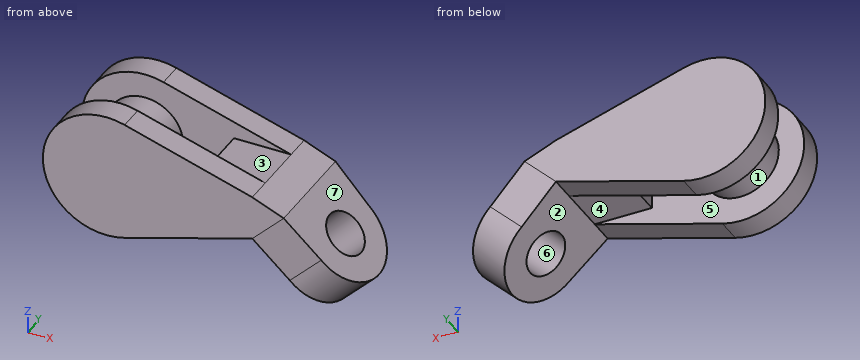
from build123d import *

# Parameters (mm, degrees)
BOSS_EXTRUDE1_DEPTH             = 35
BOSS_EXTRUDE2_START             = -40
BOSS_EXTRUDE2_DEPTH             = 80
SKETCH7_R                       = 17.5
BOSS_EXTRUDE8_DEPTH             = 35
BOSS_EXTRUDE9_REACH             = 208.04
BOSS_EXTRUDE9_DIRECTION_2_REACH = 208.04
BOSS_EXTRUDE6_DEPTH             = 20
BOSS_EXTRUDE6_DEPTH_BACK        = 20
SKETCH5_R                       = 30
BOSS_EXTRUDE10_DEPTH            = 20


with BuildPart() as part:
    # Sketch1 → Boss-Extrude1 (new body)
    with BuildSketch(Plane.XY):
        Polygon((0, -20), (70, -20), (70, 20), (0, 20), (0, 40), (100, 40), (115, 40), (115, -40), (100, -40), (0, -40), align=None)
    extrude(amount=BOSS_EXTRUDE1_DEPTH)


with BuildPart() as body_2:
    # Sketch2 → Boss-Extrude2 (new body)
    with BuildSketch(Plane(origin=(0, 0, 0), x_dir=(1, 0, 0), z_dir=(0, 1, 0)).offset(BOSS_EXTRUDE2_START)):
        Polygon((115, -35), (115, 0), (143.284271247, 28.284271247), (160.784271247, 10.784271247), align=None)
    extrude(amount=BOSS_EXTRUDE2_DEPTH)


with BuildPart() as body_3:
    # Sketch7 → Boss-Extrude8 (new body)
    with BuildSketch(Plane(origin=(57.5, 0, 57.5), x_dir=(-0.7071067811865485, 0, 0.7071067811865466), z_dir=(-0.7071067811865466, 0, -0.7071067811865485))):
        with BuildLine():
            Line((-121.317279836, 37.5), (-81.317279836, 40))
            Line((-81.317279836, 40), (-81.317279836, -40))
            Line((-81.317279836, -40), (-121.317279836, -37.5))
            ThreePointArc((-121.317279836, -37.5), (-158.817279836, 0), (-121.317279836, 37.5))
        make_face()
        with Locations((-121.317279836, 0)):
            Circle(SKETCH7_R, mode=Mode.SUBTRACT)
    extrude(amount=-BOSS_EXTRUDE8_DEPTH)


with BuildPart() as body_4:

    # Boss-Extrude9: up to this face of the body (flat: up to its plane)
    boss_extrude9_end = Plane(part.part.faces().sort_by_distance((57.5, 40, 17.5))[0])
    # Sketch9 → Boss-Extrude9 (new, up to the picked face)
    with BuildSketch(Plane(origin=(0, 0, 0), x_dir=(1, 0, 0), z_dir=(0, 1, 0)), mode=Mode.PRIVATE) as boss_extrude9_sk1:
        Polygon((139.748737342, -24.748737342), (115, 0), (115, -35), align=None)
    boss_extrude9_tool1 = split(extrude(boss_extrude9_sk1.sketch, amount=BOSS_EXTRUDE9_REACH, mode=Mode.PRIVATE), bisect_by=boss_extrude9_end, keep=Keep.BOTH, mode=Mode.PRIVATE)
    add(boss_extrude9_tool1.solids().sort_by(Axis((123.249579, 0, 19.916246), (0, 1, 0)))[0])


    # Boss-Extrude9 direction 2: up to this face of the body (flat: up to its plane)
    boss_extrude9_direction_2_end = Plane(part.part.faces().sort_by_distance((57.5, -40, 17.5))[0])
    # Sketch9 → Boss-Extrude9 direction 2 (add, up to the picked face)
    with BuildSketch(Plane(origin=(0, 0, 0), x_dir=(1, 0, 0), z_dir=(0, 1, 0)), mode=Mode.PRIVATE) as boss_extrude9_direction_2_sk1:
        Polygon((139.748737342, -24.748737342), (115, 0), (115, -35), align=None)
    boss_extrude9_direction_2_tool1 = split(extrude(boss_extrude9_direction_2_sk1.sketch, amount=-BOSS_EXTRUDE9_DIRECTION_2_REACH, mode=Mode.PRIVATE), bisect_by=boss_extrude9_direction_2_end, keep=Keep.BOTH, mode=Mode.PRIVATE)
    add(boss_extrude9_direction_2_tool1.solids().sort_by(Axis((123.249579, 0, 19.916246), (0, -1, 0)))[0])


with BuildPart() as body_4_2:
    # Sketch5 → Boss-Extrude6 (new, two sides: drawn at the far end of the back side and taken through both)
    with BuildSketch(Plane(origin=(0, 0, 0), x_dir=(1, 0, 0), z_dir=(0, 1, 0)).offset(-BOSS_EXTRUDE6_DEPTH_BACK)):
        with Locations(Location((0, -17.943234711, 0), (0, 0, 270))):
            Circle(SKETCH5_R)
    extrude(amount=BOSS_EXTRUDE6_DEPTH + BOSS_EXTRUDE6_DEPTH_BACK)


with BuildPart() as body_5:
    # Sketch6 → Boss-Extrude10 (new body)
    with BuildSketch(Plane(origin=(0, 20, 0), x_dir=(1, 0, 0), z_dir=(0, 1, 0))):
        with BuildLine():
            Line((115, -35), (46.837484988, -35))
            ThreePointArc((46.837484988, -35), (50, -17.5), (46.837484988, 0))
            Line((46.837484988, 0), (115, 0))
            Line((115, 0), (14.455350542, 30.364839295))
            ThreePointArc((14.455350542, 30.364839295), (-50, -17.5), (14.455350542, -65.364839295))
            Line((14.455350542, -65.364839295), (115, -35))
        make_face()
    extrude(amount=BOSS_EXTRUDE10_DEPTH)


with BuildPart() as body_6:
    # Body-Move/Copy2: copy of body 5
    add(body_5.part.moved(Location((0, -60, 0))))


with BuildPart() as body_5_1:
    add(body_5.part)

    # Combine1: union part, body 4, body 3, body 6, body 4 2
    add(part.part)
    add(body_4.part)
    add(body_3.part)
    add(body_6.part)
    add(body_4_2.part)


solid = body_5_1.part
Verification items for the finished model (mm, model axes). Face numbers are marked on the shaded views. A direction names the side the tool comes from. Coordinates: 2 decimals unless noted, no trailing zeros. Write each loop counter-clockwise with the first axis right and the second up, starting at its lowest first coordinate (ties: lowest second). Pieces come first, ordered by that corner, then holes. Notation, with made-up numbers: (69, 51.25) -> (127, 51.25) arc R23 ccw to (127, 86.25) -> close; hole circle Ø2 at (58, 19.25). An arc over 180 degrees is marked (long way). One line per item, written item: value. Start each with the question number.
Q1. Access from +Z, -Z, +X, -X, +Y, -Y to the whole of each face (thin tool, end or side, straight path). Record for the marked faces 1, 2, 3 and 4.
Q2. Go/stop test with flat-tipped pins: P1, Ø2, axis at y = -29, z = -19.5, coming from the +X side; P2, Ø17.5, axis at y = -6, z = 16.5, coming from the -X side; P3, Ø20, axis at x = 103, y = 1, coming from the -Z side. Record where each tip stops, or that it passes through.
Q3. Cross-section at C-C on x = 60.5. Enter the section's corners in (y, z).
Q4. Cross-section at A-A on y = -6. Enter the section's corners in (x, z), and give its area (3 significant figures).
Q5. Mould release check, pull along Z, two halves, no side actions. Record for the marked faces 5, 6 and 7: pulls with the +Z half, pulls with the -Z half, needs draft (parallel to the pull), parting line crosses it, or undercut.
Q6. Cross-section at D-D on x = 0. Enter the section's corners in (y, z).
Q7. Thickness scan on L1, parallel to Y at x = 63, z = 32; L2, parallel to X at y = -5, z = 5; L3, parallel to Y at x = 157.5, z = 0.5. Record the ranges inside material, lowest first. Write a range as from..to.
Q8. Cross-section at B-B on z = 18. Enter the section's corners in (x, y).
Checked values:
1. face 1: none
1. face 2: -Z, +Y, -Y
1. face 3: +Z, +X
1. face 4: -Z
2. P1: stops at x = 184.98
2. P2: stops at x = -30
2. P3: stops at z = 0
3. outline: (-40, -16.46) -> (-20, -16.46) -> (-20, 51.46) -> (-40, 51.46) -> close; (20, -16.46) -> (40, -16.46) -> (40, 51.46) -> (20, 51.46) -> close
4. outline: circle Ø60 at (0, 17.94); (70, 0) -> (115, 0) -> (131.66, -16.66) -> (156.41, 8.09) -> (139.75, 24.75) -> (115, 35) -> (70, 35) -> close; (154.91, -39.91) -> (169.46, -54.46) -> (194.21, -29.71) -> (179.66, -15.16) -> close
4. area: 6,380 mm²
5. face 5: needs draft
5. face 6: undercut
5. face 7: pulls with the +Z half
6. outline: (-40, -32.5) -> (-20, -32.5) -> (-20, -12.06) -> (20, -12.06) -> (20, -32.5) -> (40, -32.5) -> (40, 67.5) -> (20, 67.5) -> (20, 47.94) -> (-20, 47.94) -> (-20, 67.5) -> (-40, 67.5) -> close
7. L1: y = -40..-20, 20..40
7. L2: x = -27.06..27.06, 70..152.85
7. L3: y = -38.14..-14.15, 14.15..38.14
8. outline: (-50, -40) -> (133, -40) -> (146.5, -39.4) -> (146.5, 39.4) -> (133, 40) -> (-50, 40) -> (-50, 20) -> (-30, 20) -> (-30, -20) -> (-50, -20) -> close; hole (30, -20) -> (70, -20) -> (70, 20) -> (30, 20) -> close
